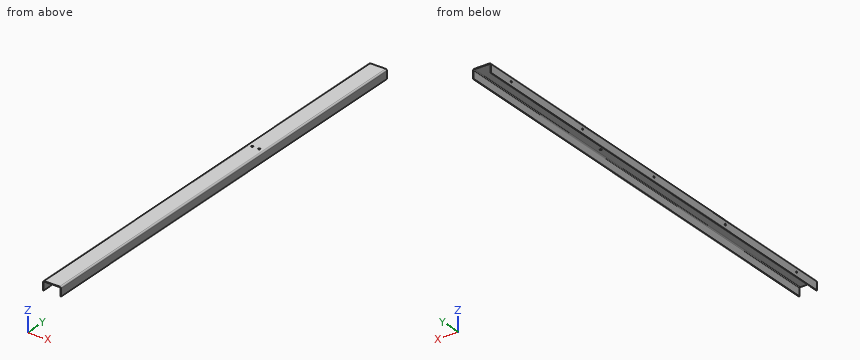
from build123d import *

# Parameters (mm, degrees)
SM_BASE_FLANGE_1_DEPTH      = 800
HOLE_WIZARD_5_5_5_5_1_D     = 5.5
HOLE_WIZARD_5_5_5_5_1_DEPTH = 2
HOLE_WIZARD_6_5_6_5_1_D     = 6.5


# Sheet-metal steps are written as plain solids
with BuildPart() as part:
    # Sketch 1 → 基体-法兰1 (new, symmetric)
    with BuildSketch(Plane(origin=(0, 0, 0), x_dir=(1, 0, 0), z_dir=(0, 1, 0))):
        with BuildLine():
            Line((-30, 30), (-30, 3))
            ThreePointArc((-30, 3), (-29.121320344, 0.878679656), (-27, 0))
            Line((-27, 0), (27, 0))
            ThreePointArc((27, 0), (29.121320344, 0.878679656), (30, 3))
            Line((30, 3), (30, 30))
            Line((30, 30), (32, 30))
            Line((32, 30), (32, 3))
            ThreePointArc((32, 3), (30.535533906, -0.535533906), (27, -2))
            Line((27, -2), (-27, -2))
            ThreePointArc((-27, -2), (-30.535533906, -0.535533906), (-32, 3))
            Line((-32, 3), (-32, 30))
            Line((-32, 30), (-30, 30))
        make_face()
    extrude(amount=SM_BASE_FLANGE_1_DEPTH, both=True)

    # Ø5.5 (5.5) 直径孔1
    with Locations(Plane(origin=(-32, 700, -15), x_dir=(0, 0, -1), z_dir=(-1, 0, 0))):
        with Locations((0, 0), (0, 350), (0, 700), (0, 1050), (0, 1400)):
            Hole(HOLE_WIZARD_5_5_5_5_1_D / 2, depth=HOLE_WIZARD_5_5_5_5_1_DEPTH)

    # Ø6.5 (6.5) 直径孔1 (through all)
    with Locations(Plane(origin=(-12.5, 200, 0), x_dir=(-1, 0, 0), z_dir=(0, 0, -1))):
        with Locations((0, 0), (-25, 0)):
            Hole(HOLE_WIZARD_6_5_6_5_1_D / 2)


solid = part.part
Can you work these out from the model? Positions are in its coordinate system, mm. Coordinates: 2 decimals unless noted, no trailing zeros. Order: outer loops, then holes, each group sorted by start corner. A loop starts at its lowest first (then second) coordinate and runs counter-clockwise, first axis right, second up. Notation, with made-up numbers: M 26,-12.5 L 35,-12.5 A37 ccw 35,26.5 Z; hole C 68,-35.5 d1. An arc over 180 degrees is marked long. Write item = value, one per line.
(1) I need wall thicknesses on line 1 along Y through (x, z) = (-31, -15); line 2 along X through (y, z) = (200, 0.85); line 3 along X through (y, z) = (588, -19). Which ranges of each line are inside material? Lowest first, please. Write a range as [from, to].
Results are:
line_1 = [-800, -702.75], [-697.25, -352.75], [-347.25, -2.75], [2.75, 347.25], [352.75, 697.25], [702.75, 800]
line_2 = [-30.19, -15.75], [-9.25, 9.25], [15.75, 30.19]
line_3 = [-32, -30], [30, 32]
(2) Suppose I cut it at A-A on y = -434. Please give me the cut outline in (x, z), plus the area to 3 significant figures.
Results are:
outline = M -32,-30 L -30,-30 L -30,-3 A3 cw -27,0 L 27,0 A3 cw 30,-3 L 30,-30 L 32,-30 L 32,-3 A5 ccw 27,2 L -27,2 A5 ccw -32,-3 Z
area = 241 mm2
(3) For pin 1 Ø8.5 at (x, y) = (12.5, 200) entering from -Z; pin 2 Ø8 at (x, y) = (24.5, -424.5) entering from -Z, each with a flat end and sliding along its axis, tell me the tip position at first contact or that it passes through.
Results are:
pin_1 = 0
pin_2 = -0.4
